The model under review builds one solid part; all positions refer to its coordinate system, in mm. Face numbers are marked on the shaded views. A direction names the side the tool comes from. Round coordinates to 2 decimals unless told otherwise and drop trailing zeros. Order: outer loops, then holes, each group sorted by start corner. A loop starts at its lowest first (then second) coordinate and runs counter-clockwise, first axis right, second up.
1) Consider section B-B (z = 30). Give the boundary of the cut face in (x, y), then the cut area to 3 significant figures.
2) Clearance check with flat-ended pins moving along their axes: P1, Ø12, axis at x = -51, y = 58, coming from the +Z side; P2, Ø1.5, axis at x = 17.5, y = 152, coming from the +Z side; P3, Ø1.5, axis at x = 66.5, y = 61.5, coming from the -Z side. State where each tip first meets the part, or that it passes through.
3) Consider section D-D (y = 132.5). Give the boundary of the cut face in (x, z), then the cut area to 3 significant figures.
4) Machinability: for the marked faces 4 and 5, which of the approach directions +Z, -Z, +X, -X, +Y, -Y give a long, thin tool a straight path to every point of the face, cutting with its end or side? Answer none if there is none.
5) Consider section A-A (y = 76). Give the boundary of the cut face in (x, z).
6) Consider section C-C (x = 47.5). Give the boundary of the cut face in (y, z).
7) To check wall thickness, follow L1, parallel to Y at x = -68, z = -17; L2, parallel to X at y = 117, z = -12.5; L3, parallel to X at y = 34.5, z = -1. State the ranges of each line that lie inside material, in increasing order.
8) Mouldability with a two-part tool opening along X and no side actions: class the marked faces 1, 2 and 3 as pulls with the +X half, pulls with the -X half, needs draft (parallel to the pull), parting line crosses it, or undercut.
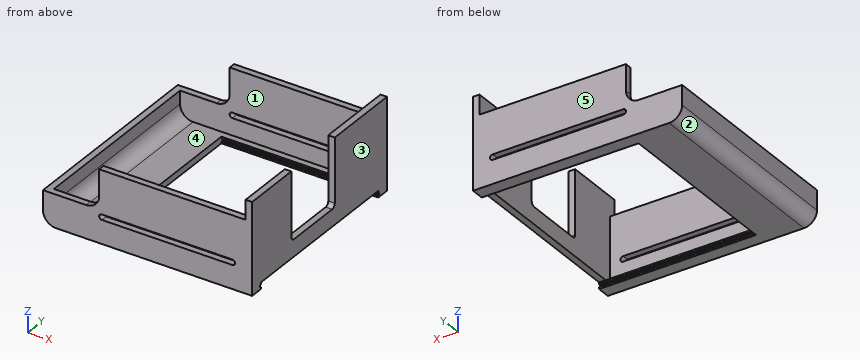
from build123d import *

# Parameters (mm, degrees)
BOSS_EXTRUDE1_DEPTH = 5
SKETCH2_W           = 150
SKETCH2_H           = 5
BOSS_EXTRUDE2_DEPTH = 145
SKETCH6_W           = 70
SKETCH6_H           = 155
BOSS_EXTRUDE3_DEPTH = 5
SKETCH7_W           = 52
SKETCH7_H           = 50
CUT_EXTRUDE1_DEPTH  = 5
SKETCH8_W           = 25
SKETCH8_H           = 155
BOSS_EXTRUDE4_DEPTH = 5
FILLET1_R           = 10
FILLET2_R           = 10
SKETCH9_W           = 2
SKETCH9_H           = 1
CUT_EXTRUDE2_DEPTH  = 120
FILLET5_R           = 3
CUT_EXTRUDE4_START  = -155
CUT_EXTRUDE4_DEPTH  = 155


with BuildPart() as part:
    # Sketch1 → Boss-Extrude1 (new body)
    with BuildSketch(Plane(origin=(0, 0, 0), x_dir=(1, 0, 0), z_dir=(0, 1, 0))):
        Polygon((63.462686567, 36.156716418), (-86.537313433, 36.156716418), (-86.537313433, 11.156716418), (-48.537313433, 11.156716418), (-48.537313433, -18.843283582), (63.462686567, -18.843283582), align=None)
    boss_extrude1 = extrude(amount=BOSS_EXTRUDE1_DEPTH)

    # Sketch2 → Boss-Extrude2 (add)
    with BuildSketch(Plane(origin=(0, 5, 0), x_dir=(1, 0, 0), z_dir=(0, 1, 0))):
        with Locations((-11.537313433, 33.656716418)):
            Rectangle(SKETCH2_W, SKETCH2_H)
    extrude(amount=BOSS_EXTRUDE2_DEPTH)

    # Mirror1: Boss-Extrude1 across plane
    add(boss_extrude1.mirror(Plane.ZX.offset(77.5)))

    # Sketch6 → Boss-Extrude3 (add)
    with BuildSketch(Plane(origin=(63.462686567, 0, 0), x_dir=(0, 0, -1), z_dir=(1, 0, 0))):
        with Locations((1.156716418, 77.5)):
            Rectangle(SKETCH6_W, SKETCH6_H)
    extrude(amount=BOSS_EXTRUDE3_DEPTH)

    # Sketch7 → Cut-Extrude1 (cut)
    with BuildSketch(Plane(origin=(68.462686567, 0, 0), x_dir=(0, 0, -1), z_dir=(1, 0, 0))):
        with Locations((-7.843283582, 70)):
            Rectangle(SKETCH7_W, SKETCH7_H)
    extrude(amount=-CUT_EXTRUDE1_DEPTH, mode=Mode.SUBTRACT)

    # Sketch8 → Boss-Extrude4 (add)
    with BuildSketch(Plane.ZY.offset(86.537313433)):
        with Locations((-23.656716418, 77.5)):
            Rectangle(SKETCH8_W, SKETCH8_H)
    extrude(amount=BOSS_EXTRUDE4_DEPTH)

    # Fillet1
    fillet1_edges = [part.edges().sort_by_distance(p)[0] for p in [
        (-48.537313433, 2.5, -11.156716418),
        (-48.537313433, 152.5, -11.156716418),
        (-91.537313433, 77.5, -36.156716418),
    ]]
    fillet(fillet1_edges, radius=FILLET1_R)

    # Fillet2
    fillet2_edges = [part.edges().sort_by_distance(p)[0] for p in [
        (-86.537313433, 77.5, -31.156716418),
    ]]
    fillet(fillet2_edges, radius=FILLET2_R)

    # Sketch9 → Cut-Extrude2 (cut)
    with BuildSketch(Plane(origin=(68.462686567, 0, 0), x_dir=(0, 0, -1), z_dir=(1, 0, 0))):
        Polygon((36.156716418, 10), (36.156716418, 145), (34.656716418, 145), (32.656716418, 145), (31.156716418, 145), (31.156716418, 10), (32.656716418, 10), (34.656716418, 10), align=None)
        with Locations((33.656716418, 9.5)):
            Rectangle(SKETCH9_W, SKETCH9_H)
        with Locations((33.656716418, 145.5)):
            Rectangle(SKETCH9_W, SKETCH9_H)
    extrude(amount=-CUT_EXTRUDE2_DEPTH, mode=Mode.SUBTRACT)

    # Fillet5
    fillet5_edges = [part.edges().sort_by_distance(p)[0] for p in [
        (65.962686567, 95, -18.156716418),
        (65.962686567, 45, -18.156716418),
    ]]
    fillet(fillet5_edges, radius=FILLET5_R)

    # Sketch11 → Cut-Extrude4 (cut)
    with BuildSketch(Plane.XZ.offset(CUT_EXTRUDE4_START)):
        with BuildLine():
            Line((53.462686567, -18.206716418), (-46.537313433, -18.206716418))
            ThreePointArc((-46.537313433, -18.206716418), (-48.587313433, -16.156716418), (-46.537313433, -14.106716418))
            Line((-46.537313433, -14.106716418), (53.462686567, -14.106716418))
            ThreePointArc((53.462686567, -14.106716418), (55.512686567, -16.156716418), (53.462686567, -18.206716418))
        make_face()
    extrude(amount=CUT_EXTRUDE4_DEPTH, mode=Mode.SUBTRACT)


solid = part.part
Answer below:
1. outline: (63.46, 0) - (68.46, 0) - (68.46, 45) - (63.46, 45) - close; (63.46, 95) - (68.46, 95) - (68.46, 155) - (63.46, 155) - close
1. area: 525 mm2
2. P1: stops at z = -31.16
2. P2: stops at z = 18.84
2. P3: stops at z = -31.16
3. outline: (-91.54, -26.16) arc R10 ccw to (-81.54, -36.16) - (-51.54, -36.16) - (-51.54, -31.16) - (-76.54, -31.16) arc R10 cw to (-86.54, -21.16) - (-86.54, -11.16) - (-91.54, -11.16) - close; (63.46, -31.16) - (68.46, -31.16) - (68.46, 33.84) - (63.46, 33.84) - close
3. area: 625 mm2
4. face 4: +Z
4. face 5: +Z, -Z, +X, -X, +Y
5. outline: (-91.54, -26.16) arc R10 ccw to (-81.54, -36.16) - (-51.54, -36.16) - (-51.54, -31.16) - (-76.54, -31.16) arc R10 cw to (-86.54, -21.16) - (-86.54, -11.16) - (-91.54, -11.16) - close; (63.46, -31.16) - (68.46, -31.16) - (68.46, -18.16) - (63.46, -18.16) - close
6. outline: (0, -36.16) - (10, -36.16) - (10, -34.66) - (9, -34.66) - (9, -32.66) - (10, -32.66) - (10, -31.16) - (5, -31.16) - (5, -18.21) - (0, -18.21) - close; (0, -14.11) - (5, -14.11) - (5, 18.84) - (0, 18.84) - close; (145, -36.16) - (155, -36.16) - (155, -18.21) - (150, -18.21) - (150, -31.16) - (145, -31.16) - (145, -32.66) - (146, -32.66) - (146, -34.66) - (145, -34.66) - close; (150, -14.11) - (155, -14.11) - (155, 18.84) - (150, 18.84) - close
7. L1: y = 0 to 5, 150 to 155
7. L2: x = -91.54 to -86.54, 63.46 to 68.46
7. L3: x = 63.46 to 68.46
8. face 1: undercut
8. face 2: pulls with the -X half
8. face 3: pulls with the +X half
